from build123d import *

# Parameters (mm, degrees)
BOSS_EXTRUDE1_DEPTH = 35
FILLET1_R           = 5
CUT_EXTRUDE1_REACH  = 61.592
SKETCH2_R           = 4.1


with BuildPart() as part:
    # Sketch1 → Boss-Extrude1 (new body)
    with BuildSketch(Plane(origin=(0, 0, 0), x_dir=(1, 0, 0), z_dir=(0, 1, 0))):
        with BuildLine():
            ThreePointArc((-35, -12), (-40.674548662, -10.573528147), (-45, -6.633249581))
            Line((-45, -6.633249581), (-47.5, -8.291561976))
            ThreePointArc((-47.5, -8.291561976), (-42.093185827, -13.216910184), (-35, -15))
            Line((-35, -15), (35, -15))
            ThreePointArc((35, -15), (42.093185827, -13.216910184), (47.5, -8.291561976))
            Line((47.5, -8.291561976), (45, -6.633249581))
            ThreePointArc((45, -6.633249581), (40.674548662, -10.573528147), (35, -12))
            Line((35, -12), (-35, -12))
        make_face()
    extrude(amount=BOSS_EXTRUDE1_DEPTH)

    # Fillet1
    fillet1_edges = [part.edges().sort_by_distance(p)[0] for p in [
        (46.25, 0, 7.462405778),
        (-46.25, 0, 7.462405778),
        (46.25, 35, 7.462405778),
        (-46.25, 35, 7.462405778),
    ]]
    fillet(fillet1_edges, radius=FILLET1_R)

    # Sketch2 → Cut-Extrude1 (cut, up to next)
    with BuildSketch(Plane.XY.offset(15), mode=Mode.PRIVATE) as cut_extrude1_sk1:
        with Locations((0, 17.5)):
            Circle(SKETCH2_R)
    cut_extrude1_tool1 = extrude(cut_extrude1_sk1.sketch, amount=-CUT_EXTRUDE1_REACH, mode=Mode.PRIVATE) & part.part
    add(cut_extrude1_tool1.solids().sort_by_distance((0, 17.5, 15))[0], mode=Mode.SUBTRACT)


solid = part.part
Input: part model. Units: mm. Frame: model coordinates. A direction names the side the tool comes from. Coordinates: 2 decimals unless noted, no trailing zeros. Loops run counter-clockwise (first coordinate to the right, second up) from the corner with the lowest first, then second, coordinate; pieces in that order, holes last. Notation, with made-up numbers: (86.25, -23) -> (136.25, -23) arc R16 ccw to (136.25, -13) -> close; hole circle Ø6 at (20, 71). An arc over 180 degrees is marked (long way). One line per item, written item: value.
(1) Ray query, line 1 along Y through (x, z) = (0, 13); line 2 along Z through (x, y) = (30, 10.5); line 3 along X through (y, z) = (26, 10). Return the intervals inside material, ascending.
Answer below:
line 1: y = 0 to 13.4, 21.6 to 35
line 2: z = 12 to 15
line 3: x = -46.18 to -41.63, 41.63 to 46.18
(2) Cut plane A-A (x = 0). Output: boundary loops of the cut face in (y, z).
Answer below:
outline: (0, 12) -> (13.4, 12) -> (13.4, 15) -> (0, 15) -> close; (21.6, 12) -> (35, 12) -> (35, 15) -> (21.6, 15) -> close
(3) Cut plane C-C (y = 10). Output: boundary loops of the cut face in (x, z), then the cut area to 3 significant figures.
Answer below:
outline: (-47.5, 8.29) -> (-45, 6.63) arc R12 cw to (-35, 12) -> (35, 12) arc R12 cw to (45, 6.63) -> (47.5, 8.29) arc R15 ccw to (35, 15) -> (-35, 15) arc R15 ccw to start
area: 290 mm2
(4) Cut plane B-B (y = 17.5). Output: boundary loops of the cut face in (x, z).
Answer below:
outline: (-47.5, 8.29) -> (-45, 6.63) arc R12 cw to (-35, 12) -> (-4.1, 12) -> (-4.1, 15) -> (-35, 15) arc R15 ccw to start; (4.1, 12) -> (35, 12) arc R12 cw to (45, 6.63) -> (47.5, 8.29) arc R15 ccw to (35, 15) -> (4.1, 15) -> close
(5) Cut plane D-D (x = -32). Output: boundary loops of the cut face in (y, z), then the cut area to 3 significant figures.
Answer below:
outline: (0, 12) -> (35, 12) -> (35, 15) -> (0, 15) -> close
area: 105 mm2
(6) Draft query along X for faces 3 (the face through (45.362, 1.504, 8.584)), 4 (the face through (-1, 35, 13)), 5 (the face through (40.747, 17.255, 10.534)). Return one class per face: pulls with the +X half, pulls with the -X half, needs draft (parallel to the pull), parting line crosses it, or undercut.
Answer below:
face 3: pulls with the +X half
face 4: needs draft
face 5: undercut
(7) Set-up query: faces 1 (the face through (-40.602, 17.255, 10.612)), 2 (the face through (-46.23, 17.32, 7.45)). Return all of +Z, -Z, +X, -X, +Y, -Y with unobstructed straight access to the full face (end or side cutting, diameter ignored); none if empty.
Answer below:
face 1: -Z, +Y, -Y
face 2: -Z, -X, +Y, -Y
(8) Pin query (flat end, axial travel): pin 1 Ø3 at (x, y) = (-15.5, 22.5) entering from -Z; pin 2 Ø1 at (y, z) = (29.5, 12) entering from -X; pin 3 Ø1 at (y, z) = (9.5, 9.5) entering from +X. Return the tip coordinate at first contact, or that it passes through.
Answer below:
pin 1: stops at z = 12
pin 2: stops at x = -44.63
pin 3: stops at x = 47
